Geometry check sheet. Reference: the model listing, model coordinates, mm. A direction names the side the tool comes from. Coordinates: 2 decimals unless noted, no trailing zeros. Write each loop counter-clockwise with the first axis right and the second up, starting at its lowest first coordinate (ties: lowest second). Pieces come first, ordered by that corner, then holes. Notation, with made-up numbers: M 14.5,-15 L 41.5,-15 A15 cw 41.5,1 Z; hole C 67.25,-7 d10. An arc over 180 degrees is marked long. Write each question's results on one line, items separated by ' | '.
```python
from build123d import *

# Parameters (mm, degrees)
SKETCH1_W           = 20
SKETCH1_H           = 50
BOSS_EXTRUDE1_DEPTH = 50
SKETCH2_R           = 5
BOSS_EXTRUDE2_DEPTH = 5
SKETCH3_R           = 2.5
CUT_EXTRUDE1_DEPTH  = 5
FILLET1_R           = 1


with BuildPart() as part:
    # Sketch1 → Boss-Extrude1 (new body)
    with BuildSketch(Plane(origin=(0, 0, 0), x_dir=(1, 0, 0), z_dir=(0, 1, 0))):
        Rectangle(SKETCH1_W, SKETCH1_H)
    extrude(amount=BOSS_EXTRUDE1_DEPTH)

    # Sketch2 → Boss-Extrude2 (add)
    with BuildSketch(Plane(origin=(0, 50, 0), x_dir=(1, 0, 0), z_dir=(0, 1, 0))):
        with Locations(Location((0, 15, 0), (0, 0, 270))):
            Circle(SKETCH2_R)
    extrude(amount=BOSS_EXTRUDE2_DEPTH)

    # Sketch3 → Cut-Extrude1 (cut)
    with BuildSketch(Plane(origin=(0, 55, 0), x_dir=(1, 0, 0), z_dir=(0, 1, 0))):
        with Locations(Location((0, 15, 0), (0, 0, 270))):
            Circle(SKETCH3_R)
    extrude(amount=-CUT_EXTRUDE1_DEPTH, mode=Mode.SUBTRACT)

    # Fillet1
    fillet1_edges = [part.edges().sort_by_distance(p)[0] for p in [
        (0, 55, -20),
    ]]
    fillet(fillet1_edges, radius=FILLET1_R)


solid = part.part
```
Q1. Sectioned sample at A-A on x = 0. Record the cut outline in (y, z).
Geometry check:
outline: M 0,-25 L 50,-25 L 50,-20 L 54,-20 A1 ccw 55,-19 L 55,-17.5 L 50,-17.5 L 50,-12.5 L 55,-12.5 L 55,-11 A1 ccw 54,-10 L 50,-10 L 50,25 L 0,25 Z
Q2. Depth check by flat-ended pin: P1, Ø2, axis at x = -6, z = 14, coming from the +Y side. Enter the tip coordinate at first touch or a pass-through.
Geometry check:
P1: stops at y = 50
Q3. Access from +Z, -Z, +X, -X, +Y, -Y to the whole of each face (thin tool, end or side, straight path). Record for faces 4 (the flat face through (10, 25, 0)), 5 (the cylindrical face through (0.1, 52.5, -17.5)).
Geometry check:
face 4: +Z, -Z, +X, +Y, -Y | face 5: +Y
Q4. Mould release check, pull along X, two halves, no side actions. Record for faces 1 (the cylindrical face through (0, 52, -20)), 2 (the flat face through (0, 50, -15)), 3 (the flat face through (-2, 55, -17)): pulls with the +X half, pulls with the -X half, needs draft (parallel to the pull), parting line crosses it, or undercut.
Geometry check:
face 1: parting line crosses it | face 2: undercut | face 3: needs draft
Q5. Sectioned sample at B-B on z = -15. Record the cut outline in (x, y).
Geometry check:
outline: M -10,0 L 10,0 L 10,50 L 5,50 L 5,54 A1 ccw 4,55 L 2.5,55 L 2.5,50 L -2.5,50 L -2.5,55 L -4,55 A1 ccw -5,54 L -5,50 L -10,50 Z
Q6. Sectioned sample at D-D on z = -0.5. Record the cut outline in (x, y), and give its area (3 significant figures).
Geometry check:
outline: M -10,0 L 10,0 L 10,50 L -10,50 Z | area: 1,000 mm2
Q7. Sectioned sample at C-C on x = 6.75. Record the cut outline in (y, z), and give its area (3 significant figures).
Geometry check:
outline: M 0,-25 L 50,-25 L 50,25 L 0,25 Z | area: 2,500 mm2
Q8. Scan lines: probe 1 along X at (y, z) = (53.3, -15); probe 2 along Y at (x, z) = (7.5, -0.5). Record each from-to range of solid material in increasing order.
Geometry check:
probe 1: x = -5 to -2.5, 2.5 to 5 | probe 2: y = 0 to 50
